CAD build for the part. Positions are in the model's coordinates, mm. A direction names the side the tool comes from. Give positions to 0.01 mm unless a question says otherwise; leave off trailing zeros. Order: outer loops, then holes, each group sorted by start corner. A loop starts at its lowest first (then second) coordinate and runs counter-clockwise, first axis right, second up.
Item 1: Band-saw the part on B-B on z = 6. Give the cut face in (x, y), plus the area to 3 significant figures.
Item 2: Two-plate mould, pull along X, no slides. Class faces 1 (the flat face through (28, 2, 4)), 2 (the flat face through (71, 47, 6)), 3 (the flat face through (37, 0, 3)): released by +X, released by -X, zero draft, split by the parting line, or undercut.
Item 3: Flat gauge pins, fed straight in: P1, Ø3, axis at y = 13.5, z = 6.5, coming from the -X side; P2, Ø3, axis at x = 27.5, z = 4.5, coming from the +Y side; P3, Ø3, axis at y = 52.5, z = 1.5, coming from the -X side. Where does each tip first touch, or does it go through?
Item 4: Wall check: L1, parallel to Y at x = 50.5, z = 3; L2, parallel to Y at x = 30, z = 1.75; L3, parallel to X at y = 48, z = 4. Give the ranges that are in metal, low to high.
Item 5: Which spindle directions (+Z, -Z, +X, -X, +Y, -Y) get a long thin tool onto all of the face, cutting with end or side? Do faces 4 (the flat face through (65.577, 20.238, 5.916)), 5 (the flat face through (60, 59, 4)), 6 (the cylindrical face through (6, 2, 6)), 7 (the cylindrical face through (50, 2, 6)). Say none if no direction does.
Item 6: Band-saw the part on C-C on x = 62.5. Give the cut face in (y, z), plus the area to 3 significant figures.
Item 7: Band-saw the part on A-A on x = 43. Give the cut face in (y, z).
Item 8: Band-saw the part on D-D on y = 56. Give the cut face in (x, z), plus the area to 3 significant figures.
```python
from build123d import *

# Parameters (mm, degrees)
PAD_DEPTH       = 12
POCKET_DEPTH    = 5
POCKET001_DEPTH = 5


with BuildPart() as part:
    # Sketch → Pad (new body)
    with BuildSketch(Plane.XY):
        Polygon((0, 0), (76, 0), (76, 60), (46, 60), (46, 57), (71, 57), (71, 37), (60, 3), (0, 3), align=None)
    extrude(amount=PAD_DEPTH)

    # Sketch001 (on Face3 of Pad) → Pocket (cut)
    with BuildSketch(Plane(origin=(0, 60, 0), x_dir=(-1, 0, 0), z_dir=(0, 1, 0))):
        with BuildLine():
            ThreePointArc((-67, 8), (-69, 6), (-67, 4))
            Line((-67, 4), (-53, 4))
            ThreePointArc((-53, 4), (-51, 6), (-53, 8))
            Line((-53, 8), (-67, 8))
        make_face()
    extrude(amount=-POCKET_DEPTH, mode=Mode.SUBTRACT)

    # Sketch002 (on Face6 of Pocket) → Pocket001 (cut)
    with BuildSketch(Plane(origin=(0, 3, 0), x_dir=(-1, 0, 0), z_dir=(0, 1, 0))):
        with BuildLine():
            ThreePointArc((-48, 8), (-50, 6), (-48, 4))
            Line((-48, 4), (-8, 4))
            ThreePointArc((-8, 4), (-6, 6), (-8, 8))
            Line((-48, 8), (-8, 8))
        make_face()
    extrude(amount=-POCKET001_DEPTH, mode=Mode.SUBTRACT)


solid = part.part
```
The answers:
1. outline: (0, 0) - (6, 0) - (6, 3) - (0, 3) - close; (46, 57) - (51, 57) - (51, 60) - (46, 60) - close; (50, 0) - (76, 0) - (76, 60) - (69, 60) - (69, 57) - (71, 57) - (71, 37) - (60, 3) - (50, 3) - close
1. area: 589 mm2
2. face 1: undercut
2. face 2: released by -X
2. face 3: zero draft
3. P1: stops at x = 62.91
3. P2: stops at y = 3
3. P3: stops at x = 71
4. L1: y = 0 to 3, 57 to 60
4. L2: y = 0 to 3
4. L3: x = 71 to 76
5. face 4: +Z, -Z, -X
5. face 5: +Y
5. face 6: +Y, -Y
5. face 7: -Y
6. outline: (0, 0) - (10.73, 0) - (10.73, 12) - (0, 12) - close; (57, 0) - (60, 0) - (60, 4) - (57, 4) - close; (57, 8) - (60, 8) - (60, 12) - (57, 12) - close
6. area: 153 mm2
7. outline: (0, 0) - (3, 0) - (3, 4) - (0, 4) - close; (0, 8) - (3, 8) - (3, 12) - (0, 12) - close
8. outline: (71, 0) - (76, 0) - (76, 12) - (71, 12) - close
8. area: 60.0 mm2
